Build history of the part. All positions in model axes, mm. Face numbers are marked on the shaded views. Round coordinates to 2 decimals unless told otherwise and drop trailing zeros. Write each loop counter-clockwise with the first axis right and the second up, starting at its lowest first coordinate (ties: lowest second). Pieces come first, ordered by that corner, then holes. Notation, with made-up numbers: M -38.5,68 L -6.5,68 A8 ccw -6.5,76 Z; hole C 8,5 d4. An arc over 180 degrees is marked long. Write item = value, one per line. Start each with the question number.
Q1. Band-saw the part on C-C on x = 82.5. Write the cut outline in (y, z), plus the area to 3 significant figures.
Q2. Drop flat-ended pins along their axis: P1, Ø6, axis at x = 67, y = 26, coming from the +Z side; P2, Ø8, axis at x = 81, z = 58.5, coming from the -Y side; P3, Ø8, axis at x = 75.5, y = 83, coming from the +Z side. Give the stop position or say it passes through.
Q3. Pull direction Y, two halves, no side cores. Call the marked faces 1, 2 and 3: released by +Y, released by -Y, zero draft, split by the parting line, or undercut.
Q4. Probe L1, parallel to Y at x = 70, z = 132.5; L2, parallel to Z at x = 15, y = 66.5; L3, parallel to Z at x = 83.5, y = 53.5. List the from-to ranges inside material, lowest first.
Q5. Band-saw the part on B-B on y = 13. Write the cut outline in (x, z), plus the area to 3 significant figures.
Q6. Band-saw the part on A-A on x = 43. Write the cut outline in (y, z).
```python
from build123d import *

# Parameters (mm, degrees)
BOX003_W                 = 10
BOX003_H                 = 110
BOX003_DEPTH             = 10
ARRAY001_X_COUNT         = 4
ARRAY001_X_PITCH         = 20
ARRAY001_PLACEMENT_ANGLE = 90
BOX002_W                 = 10
BOX002_H                 = 110
BOX002_DEPTH             = 10
ARRAY_X_COUNT            = 4
ARRAY_X_PITCH            = 20
BOX001_W                 = 70
BOX001_H                 = 70
BOX001_DEPTH             = 30
BOX_W                    = 90
BOX_H                    = 90
BOX_DEPTH                = 150


with BuildPart() as almenas_y:
    # Box003 → Box003 (new body)
    with BuildSketch(Plane.XY):
        with Locations((5, 55)):
            Rectangle(BOX003_W, BOX003_H)
    extrude(amount=BOX003_DEPTH)

    # Array001 X: almenas_y ×4


with BuildPart() as almenas_y_1:
    add(almenas_y.part)
    with Locations(*[(i * ARRAY001_X_PITCH, 0, 0) for i in range(1, ARRAY001_X_COUNT)]):
        add(almenas_y.part)


with BuildPart() as almenas_y_2:
    # Array001 placement: moved
    add(almenas_y_1.part.moved(Location((90, 20, 0))).rotate(Axis((90, 20, 0), (0, 0, 1)), ARRAY001_PLACEMENT_ANGLE))


with BuildPart() as obj1:
    # Box002 → Box002 (new body)
    with BuildSketch(Plane.XY):
        with Locations((5, 55)):
            Rectangle(BOX002_W, BOX002_H)
    extrude(amount=BOX002_DEPTH)

    # Array X: obj1 ×4


with BuildPart() as obj1_1:
    add(obj1.part)
    with Locations(*[(i * ARRAY_X_PITCH, 0, 0) for i in range(1, ARRAY_X_COUNT)]):
        add(obj1.part)

    # Fusion: union almenas_y
    add(almenas_y_2.part)


with BuildPart() as obj1_2:
    # Fusion placement: moved
    add(obj1_1.part.moved(Location((10, -10, 140))))


with BuildPart() as obj2:
    # Box001 → Box001 (new body)
    with BuildSketch(Plane(origin=(10, 10, 130), x_dir=(1, 0, 0), z_dir=(0, 0, 1))):
        with Locations((35, 35)):
            Rectangle(BOX001_W, BOX001_H)
    extrude(amount=BOX001_DEPTH)


with BuildPart() as torre_almenas:
    # Box → Box (new body)
    with BuildSketch(Plane.XY):
        with Locations((45, 45)):
            Rectangle(BOX_W, BOX_H)
    extrude(amount=BOX_DEPTH)

    # Cut: cut obj2
    add(obj2.part, mode=Mode.SUBTRACT)

    # Cut001: cut obj1
    add(obj1_2.part, mode=Mode.SUBTRACT)


solid = torre_almenas.part
```
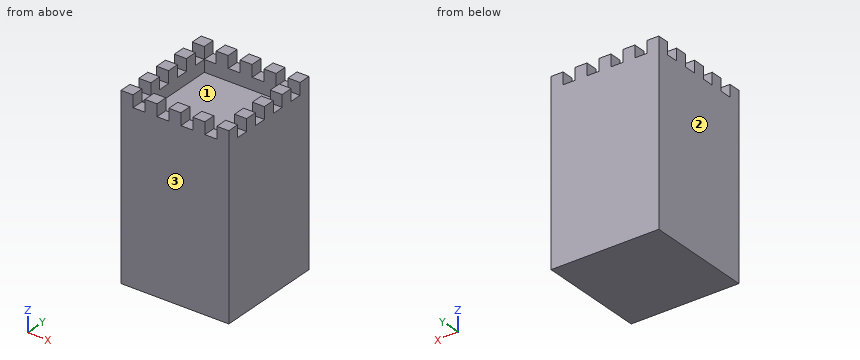
Conclusion:
q1.outline = M 0,0 L 90,0 L 90,150 L 80,150 L 80,140 L 70,140 L 70,150 L 60,150 L 60,140 L 50,140 L 50,150 L 40,150 L 40,140 L 30,140 L 30,150 L 20,150 L 20,140 L 10,140 L 10,150 L 0,150 Z
q1.area = 13,100 mm^2
q2.P1 = 130
q2.P2 = 0
q2.P3 = 140
q3.face_1 = undercut
q3.face_2 = zero draft
q3.face_3 = released by -Y
q4.L1 = 0 to 10, 80 to 90
q4.L2 = 0 to 130
q4.L3 = 0 to 140
q5.outline = M 0,0 L 90,0 L 90,140 L 80,140 L 80,130 L 10,130 L 10,140 L 0,140 Z
q5.area = 11,900 mm^2
q6.outline = M 0,0 L 90,0 L 90,150 L 80,150 L 80,130 L 10,130 L 10,150 L 0,150 Z
